Source: CAD feature listing. Evaluate the final solid. Frame: model axes, mm. Round coordinates to 2 decimals unless told otherwise and drop trailing zeros. Loops run counter-clockwise (first coordinate to the right, second up) from the corner with the lowest first, then second, coordinate; pieces in that order, holes last. Notation, with made-up numbers: (-40, -10) -> (6, -10) arc R25 cw to (6, 29) -> close; hole circle Ø6 at (85, -23.5). An arc over 180 degrees is marked (long way). Put each result on its own line as item: value. Start each with the question number.
1. Cut plane B-B (x = -27). Return the cut outline in (y, z).
2. Material intervals for L1, parallel to X at y = 2.25, z = -0.5; L2, parallel to Z at x = -27, y = 1.35; L3, parallel to Z at x = 0, y = 2.5, sorted ascending.
3. Cut plane A-A (z = 6). Return the cut outline in (x, y).
4. Draft query along X for faces 1 (the flat face through (0, 0, 0)), 2 (the cylindrical face through (-28, 2, 21)), 3 (the cylindrical face through (16.747, 1.521, 1.143)). Return one class per face: pulls with the +X half, pulls with the -X half, needs draft (parallel to the pull), parting line crosses it, or undercut.
5. Cut plane D-D (x = -13.5). Return the cut outline in (y, z), then the cut area to 3 significant figures.
6. Cut plane C-C (y = 1.85). Return the cut outline in (x, z).
```python
from build123d import *

# Parameters (mm, degrees)
SKETCH2_W          = 35
SKETCH2_H          = 3
CUT_EXTRUDE1_REACH = 51.588
SKETCH3_R          = 3.25
CUT_EXTRUDE2_REACH = 51.588
SKETCH4_R          = 2.75


with BuildPart() as part:
    # Sketch2 → Revolve1 (revolve)
    with BuildSketch(Plane.XY):
        with Locations((17.5, 1.5)):
            Rectangle(SKETCH2_W, SKETCH2_H)
    revolve(axis=Axis((0, -417.112175525, 0), (0, 1, 0)))

    # Sketch3 → Cut-Extrude1 (cut, up to next)
    with BuildSketch(Plane(origin=(0, 3, 0), x_dir=(1, 0, 0), z_dir=(0, 1, 0)), mode=Mode.PRIVATE) as cut_extrude1_sk1:
        with Locations(Location((-13.5, -1, 0), (0, 0, 180))):
            Circle(SKETCH3_R)
    cut_extrude1_tool1 = extrude(cut_extrude1_sk1.sketch, amount=-CUT_EXTRUDE1_REACH, mode=Mode.PRIVATE) & part.part
    # Sketch3 → Cut-Extrude1 (cut, up to next)
    with BuildSketch(Plane(origin=(0, 3, 0), x_dir=(1, 0, 0), z_dir=(0, 1, 0)), mode=Mode.PRIVATE) as cut_extrude1_sk2:
        with Locations(Location((13.5, -1, 0), (0, 0, 180))):
            Circle(SKETCH3_R)
    cut_extrude1_tool2 = extrude(cut_extrude1_sk2.sketch, amount=-CUT_EXTRUDE1_REACH, mode=Mode.PRIVATE) & part.part
    add(cut_extrude1_tool1.solids().sort_by_distance((-13.5, 3, 1))[0], mode=Mode.SUBTRACT)
    add(cut_extrude1_tool2.solids().sort_by_distance((13.5, 3, 1))[0], mode=Mode.SUBTRACT)

    # Sketch4 → Cut-Extrude2 (cut, up to next)
    with BuildSketch(Plane(origin=(0, 3, 0), x_dir=(1, 0, 0), z_dir=(0, 1, 0)), mode=Mode.PRIVATE) as cut_extrude2_sk1:
        with Locations(Location((-27, -7.4, 0), (0, 0, 180))):
            Circle(SKETCH4_R)
    cut_extrude2_tool1 = extrude(cut_extrude2_sk1.sketch, amount=-CUT_EXTRUDE2_REACH, mode=Mode.PRIVATE) & part.part
    # Sketch4 → Cut-Extrude2 (cut, up to next)
    with BuildSketch(Plane(origin=(0, 3, 0), x_dir=(1, 0, 0), z_dir=(0, 1, 0)), mode=Mode.PRIVATE) as cut_extrude2_sk2:
        with Locations(Location((27, -7.4, 0), (0, 0, 180))):
            Circle(SKETCH4_R)
    cut_extrude2_tool2 = extrude(cut_extrude2_sk2.sketch, amount=-CUT_EXTRUDE2_REACH, mode=Mode.PRIVATE) & part.part
    add(cut_extrude2_tool1.solids().sort_by_distance((-27, 3, 7.4))[0], mode=Mode.SUBTRACT)
    add(cut_extrude2_tool2.solids().sort_by_distance((27, 3, 7.4))[0], mode=Mode.SUBTRACT)


solid = part.part
```
Solution:
1. outline: (0, -22.27) -> (3, -22.27) -> (3, 4.65) -> (0, 4.65) -> close; (0, 10.15) -> (3, 10.15) -> (3, 22.27) -> (0, 22.27) -> close
2. L1: x = -35 to -16.38, -10.62 to 10.62, 16.38 to 35
2. L2: z = -22.27 to 4.65, 10.15 to 22.27
2. L3: z = -35 to 35
3. outline: (-34.48, 0) -> (-29.37, 0) -> (-29.37, 3) -> (-34.48, 3) -> close; (-24.63, 0) -> (24.63, 0) -> (24.63, 3) -> (-24.63, 3) -> close; (29.37, 0) -> (34.48, 0) -> (34.48, 3) -> (29.37, 3) -> close
4. face 1: needs draft
4. face 2: parting line crosses it
4. face 3: undercut
5. outline: (0, -32.29) -> (3, -32.29) -> (3, -2.25) -> (0, -2.25) -> close; (0, 4.25) -> (3, 4.25) -> (3, 32.29) -> (0, 32.29) -> close
5. area: 174 mm^2
6. outline: circle Ø70 at (0, 0); hole circle Ø5.5 at (-27, 7.4); hole circle Ø6.5 at (-13.5, 1); hole circle Ø6.5 at (13.5, 1); hole circle Ø5.5 at (27, 7.4)
